Here's how the part is built. I have some questions about the finished solid (model axes, mm). A direction names the side the tool comes from. Round coordinates to 2 decimals unless told otherwise and drop trailing zeros. Write each loop counter-clockwise with the first axis right and the second up, starting at its lowest first coordinate (ties: lowest second). Pieces come first, ordered by that corner, then holes. Notation, with made-up numbers: (82, 53.25) - (136, 53.25) arc R20 ccw to (136, 73.25) - close; hole circle Ø7 at (49, 52). An arc over 180 degrees is marked (long way). Use one line per item in the form item = value. Start each with the question number.
1. If I drill on line 1 along Y through (x, z) = (-0.65, -6.5); line 2 along Y through (x, z) = (-1.3, -12.5); line 3 along Z through (x, y) = (-0.6, -3.5), over which ranges is the centre line in solid material (lowest first)?
2. I want a section at A-A, the plane x = -2.15. State how many separate pieces and enclosed holes the cut face has, plus the area to 3 significant figures.
3. I want a section at C-C, the plane z = -2.5. List the corners of the cut face in (x, y) for me.
4. We'd pull the mould along Z, two halves only. Please class faces 4 (the conical face through (0.994, 0.123, -11.662)), 5 (the cylindrical face through (-1.532, 0.114, -12.869)), 6 (the conical face through (-1.01, 0.116, -7.214)): +Z half, -Z half, draft (parallel to the pull), parting line (faces both ways), or undercut.
5. I want a section at B-B, the plane z = -11.25. List the corners of the cut face in (x, y) for me.
6. Which directions (+Z, -Z, +X, -X, +Y, -Y) give clear straight access to the entire face, cutting with the end or side of a thin tool? Please do faces 1 (the flat face through (-1.3, 8.37, -6.7)), 2 (the cylindrical face through (-0.212, 0.118, -9.19)), 3 (the cylindrical face through (0.468, 0.121, -3.102)).
7. Will these pins go through, and if not, where does the flat tip stop? pin 1 (3 mm diameter, centred on y = 3.5, z = -7, fed in from +X); pin 2 (6 mm diameter, centred on y = -6, z = -4.5, fed in from +X); pin 3 (1.5 mm diameter, centred on x = -2, z = -1.5, fed in from +Y).
```python
from build123d import *

# Parameters (mm, degrees)
F1_ANGLE = 30


with BuildPart() as f1:
    # F0 (on Front) → F1 (revolve, symmetric)
    with BuildSketch(Plane.XZ) as f1_sk:
        Polygon((0.467722, -0.143643), (-1.532278, -0.143643), (-1.532278, -6.143643), (-1.532278, -6.417708), (-0.212138, -8.429299), (-0.212138, -9.929299), (-1.532278, -12.27802), (-1.532278, -13.443643), (-0.007577, -13.443643), (1.967722, -9.929299), (1.967722, -8.429299), (0.467722, -6.143643), align=None)
    revolve(axis=Axis((-32.532278, 0, -1.684785), (0, 0, 1)), revolution_arc=F1_ANGLE / 2)
    revolve(f1_sk.sketch, axis=Axis((-32.532278, 0, -1.684785), (0, 0, -1)), revolution_arc=F1_ANGLE / 2)


solid = f1.part
```
Model answer:
q1.line_1 = -8.54 to 8.54
q1.line_2 = -8.37 to 8.37
q1.line_3 = -13.44 to -10.28, -8.13 to -0.14
q2.separate_pieces = 4
q2.enclosed_holes = 0
q2.area = 32.4 mm2
q3.outline = (-2.59, -8.02) - (-0.66, -8.54) arc R33 ccw to (-0.66, 8.54) - (-2.59, 8.02) arc R31 cw to start
q4.face_4 = -Z half
q4.face_5 = draft
q4.face_6 = undercut
q5.outline = (-2.03, -8.17) - (0.08, -8.74) arc R33.76 ccw to (0.08, 8.74) - (-2.03, 8.17) arc R31.58 cw to start
q6.face_1 = +Z, -Z, -X, +Y
q6.face_2 = -X
q6.face_3 = +Z, +X
q7.pin_1 = 1.83
q7.pin_2 = 0.89
q7.pin_3 = 8.38
